Design review of the part built by this model. Coordinates are the model's own, in mm. Coordinates: 2 decimals unless noted, no trailing zeros. Write each loop counter-clockwise with the first axis right and the second up, starting at its lowest first coordinate (ties: lowest second). Pieces come first, ordered by that corner, then holes. Notation, with made-up numbers: (-10, -16) - (40, -16) arc R23 cw to (40, 2) - close; hole circle Ø3 at (-5.5, 39). An arc over 180 degrees is marked (long way). Use a Markdown table: item, result.
Autodesk Inventor part; units mm, degrees
ref_plane "YZ Plane" through (0, 0, 0) normal (1, 0, 0) x (0, 1, 0)
ref_plane "XZ Plane" through (0, 0, 0) normal (0, 1, 0) x (-1, 0, 0)
ref_plane "XY Plane" through (0, 0, 0) normal (0, 0, 1) x (1, 0, 0)
sketch "Szkic1" plane through (0, 0, 0) normal (0, 0, 1) x (1, 0, 0)
  circle A0 centre (0, 0) radius 5.65
  line L0 (-10.75, 1) -> (10.75, 1)
  line L1 (10.75, 1) -> (10.75, 10)
  line L2 (10.75, 10) -> (-10.75, 10)
  line L3 (-10.75, 10) -> (-10.75, 1)
  dimension "d0" = 11.3
  dimension "d1" = 21.5
  dimension "d2" = 10.75
  dimension "d3" = 1
  dimension "d4" = 9
extrude "Wyciągnięcie proste1" add sketch "Szkic1" along normal blind 12 contours L0 A0 | A0 L0 L3 L2 L1 picked at (1.0817, 2.5289)
extrude "Wyciągnięcie proste2" cut sketch "Szkic1" along normal blind 12 contours A0 L0 | L0 A0
sketch "Szkic2" plane through (10.75, 1, 0) normal (0, -1, 0) x (1, 0, 0)
  line L0 (-5.1892, 12) -> (-5.1892, 0)
  line L1 (-5.1892, 0) -> (0, 0)
  line L2 (0, 0) -> (0, 12)
  line L3 (-5.1892, 12) -> (0, 12)
  line L4 (-16.3108, 0) -> (-16.3108, 12)
  line L5 (-21.5, 12) -> (-16.3108, 12)
  line L6 (-21.5, 0) -> (-21.5, 12)
  line L7 (-21.5, 0) -> (-16.3108, 0)
  point P0 (-10.75, 0)
  point P1 (-3, 6)
  point P2 (-18.5, 6)
  dimension "d9" = 12
  dimension "d10" = 5.1892
  dimension "d11" = 3
  dimension "d12" = 6
  dimension "d13" = 6
  dimension "d14" = 3
hole "Otwór1" at (7.75, 1, 6) at (-7.75, 1, 6) direction (0, 1, 0) diameter 3 end through all
fillet "Zaokrąglenie1" radius 4 1 edges at (-10.75, 5.5, 12)
chamfer "Faza1" distance 2 angle 45 2 edges at (-10.75, 5.5, 0) (10.75, 5.5, 0)
properties part number "3DP_ABS_Induction_Sensor_Mounting_Clamp"
(1) Take a section at C-C on y = 7.5. Write out the cut boundary in (x, z), and give its area (3 significant figures).
Determined:
| item | result |
|---|---|
| outline | (-10.75, 2) - (-8.75, 0) - (8.75, 0) - (10.75, 2) - (10.75, 12) - (-6.75, 12) arc R4 ccw to (-10.75, 8) - close; hole circle Ø3 at (-7.75, 6); hole circle Ø3 at (7.75, 6) |
| area | 236 mm2 |
(2) Take a section at A-A on z = 6. Write out the cut boundary in (x, y).
Determined:
| item | result |
|---|---|
| outline | (-10.75, 1) - (-9.25, 1) - (-9.25, 10) - (-10.75, 10) - close; (-6.25, 1) - (-5.56, 1) arc R5.65 cw to (5.56, 1) - (6.25, 1) - (6.25, 10) - (-6.25, 10) - close; (9.25, 1) - (10.75, 1) - (10.75, 10) - (9.25, 10) - close |
(3) For pin 1 (1 mm diameter, centred on x = -3, y = 2, fed in from +Z), flat-tipped, find the tip position at first contact; note if it passes through.
Determined:
| item | result |
|---|---|
| pin 1 | through |
(4) Take a section at D-D on y = 4.75. Write out the cut boundary in (x, z).
Determined:
| item | result |
|---|---|
| outline | (-10.75, 2) - (-8.75, 0) - (-3.06, 0) - (-3.06, 12) - (-6.75, 12) arc R4 ccw to (-10.75, 8) - close; (3.06, 0) - (8.75, 0) - (10.75, 2) - (10.75, 12) - (3.06, 12) - close; hole circle Ø3 at (-7.75, 6); hole circle Ø3 at (7.75, 6) |
(5) Draft analysis for pull direction Z (two halves, no side actions). For faces 1 (the cylindrical face through (-6.286, 5.563, 6.325)), 2 (the cylindrical face through (9.214, 5.563, 6.325)), 3 (the flat face through (2, 7, 12)), 4 (the flat face through (-9.74, 5.44, 0.99)), state which applies: +Z half, -Z half, draft (parallel to the pull), parting line (faces both ways), or undercut.
Determined:
| item | result |
|---|---|
| face 1 | undercut |
| face 2 | undercut |
| face 3 | +Z half |
| face 4 | -Z half |
(6) Take a section at B-B on x = 7.75. Write out the cut boundary in (y, z).
Determined:
| item | result |
|---|---|
| outline | (1, 0) - (10, 0) - (10, 4.5) - (1, 4.5) - close; (1, 7.5) - (10, 7.5) - (10, 12) - (1, 12) - close |
(7) For L1, parallel to X at y = 8, z = 6; L2, parallel to Z at x = 7.75, y = 7.75; L3, parallel to X at y = 2.5, z = 3.25, list the stretches that pass through material, from the lowest coordinate up. Write a range as from..to.
Determined:
| item | result |
|---|---|
| L1 | -10.75..-9.25, -6.25..6.25, 9.25..10.75 |
| L2 | 0..4.5, 7.5..12 |
| L3 | -10.75..-5.07, 5.07..10.75 |
